from build123d import *

# Parameters (mm, degrees)
F3_R     = 12.5
F4_W     = 6
F4_H     = 10
F6_DEPTH = 8


with BuildPart() as f1:
    # F0 (on Right) → F1 (revolve)
    with BuildSketch(Plane.YZ):
        with BuildLine():
            Line((0, -25), (0, 25))
            ThreePointArc((0, 25), (-25, 0), (0, -25))
        make_face()
    revolve(axis=Axis((0, 0, 0), (0, 0, -1)))

    # F5: sweep along a path in F4
    with BuildLine(Plane.XZ) as f5_path:
        Line((25, 0), (15, 0))
        ThreePointArc((15, 0), (4.393398, -4.393398), (0, -15))
        Line((0, -15), (0, -25.968151))
    # F3 (on offset) → F5 (sweep, cut)
    with BuildSketch(Plane.YZ.offset(25)):
        Circle(F3_R)
    sweep(path=f5_path.line, mode=Mode.SUBTRACT)

    # F4 (on Front) → F6 (cut, symmetric)
    with BuildSketch(Plane.XZ):
        with Locations((-3, 20)):
            Rectangle(F4_W, F4_H)
    extrude(amount=F6_DEPTH, both=True, mode=Mode.SUBTRACT)


solid = f1.part
Can you work these out from the model? Positions are in its coordinate system, mm. A direction names the side the tool comes from. Coordinates: 2 decimals unless noted, no trailing zeros. Order: outer loops, then holes, each group sorted by start corner. A loop starts at its lowest first (then second) coordinate and runs counter-clockwise, first axis right, second up. Notation, with made-up numbers: M 73.5,20 L 93.5,20 A26 ccw 93.5,48 Z; hole C -19.5,37 d11. An arc over 180 degrees is marked long. Answer as CSV lines item,"result".
(1) I'm going to push flat-ended pins straight in: pin 1 (1.5 mm diameter, centred on x = 10.5, y = 17, fed in from -Z); pin 2 (20 mm diameter, centred on y = 0, z = 0, fed in from +X); pin 3 (5 mm diameter, centred on x = -4, z = 21.5, fed in from -Y); pin 4 (12 mm diameter, centred on x = 2.5, y = -13.5, fed in from -Z). Where does each tip first touch, or does it pass through?
Geometry check:
pin 1,"z = -15.97"
pin 2,"x = 3.54"
pin 3,"y = -15.81"
pin 4,"z = -21.65"
(2) On a 3-axis mill with a long thin cutter (end or side, diameter ignored), from which of +Z, -Z, +X, -X, +Y, -Y can I reach the whole of each face in a straight line? I mean faces 1 (the flat face through (0, 0, 20)), 2 (the cylindrical face through (18.279, 11.923, -3.755)). Say none if no direction works.
Geometry check:
face 1,"+Z"
face 2,"+X"
(3) Suppose I cut it at A-A on z = 17. Please give me the cut outline in (x, y).
Geometry check:
outline,"C 0,0 d36.66; hole M -6,-8 L 0,-8 L 0,8 L -6,8 Z"
(4) Please list where these lines run through material, in increasing order: L1, parallel to Z at x = 13, y = -1; L2, parallel to Y at x = -1, z = 3.5; L3, parallel to X at y = 3, z = -17.5.
Geometry check:
L1,"-21.33 to -13.43, 12.39 to 21.33"
L2,"-24.73 to -8.17, 8.17 to 24.73"
L3,"-17.6 to -12.13, 12.13 to 17.6"
(5) Suppose I cut it at B-B on x = -14. Please give me the cut outline in (y, z), plus the area to 3 significant figures.
Geometry check:
outline,"C 0,0 d41.42"
area,"1,350 mm^2"
